Input: dimensioned drawing with shaded views. Units: mm. Origin: part minimum x, y, z. Coordinates: 2 decimals unless noted, no trailing zeros. Loops run counter-clockwise (first coordinate to the right, second up) from the corner with the lowest first, then second, coordinate; pieces in that order, holes last. Notation, with made-up numbers: (61, -32.5) - (93, -32.5) arc R22 cw to (93, -10.5) - close; hole circle Ø11 at (-1.75, 70). An arc over 180 degrees is marked (long way). Use one line per item in the form item = value. Start each with the question number.
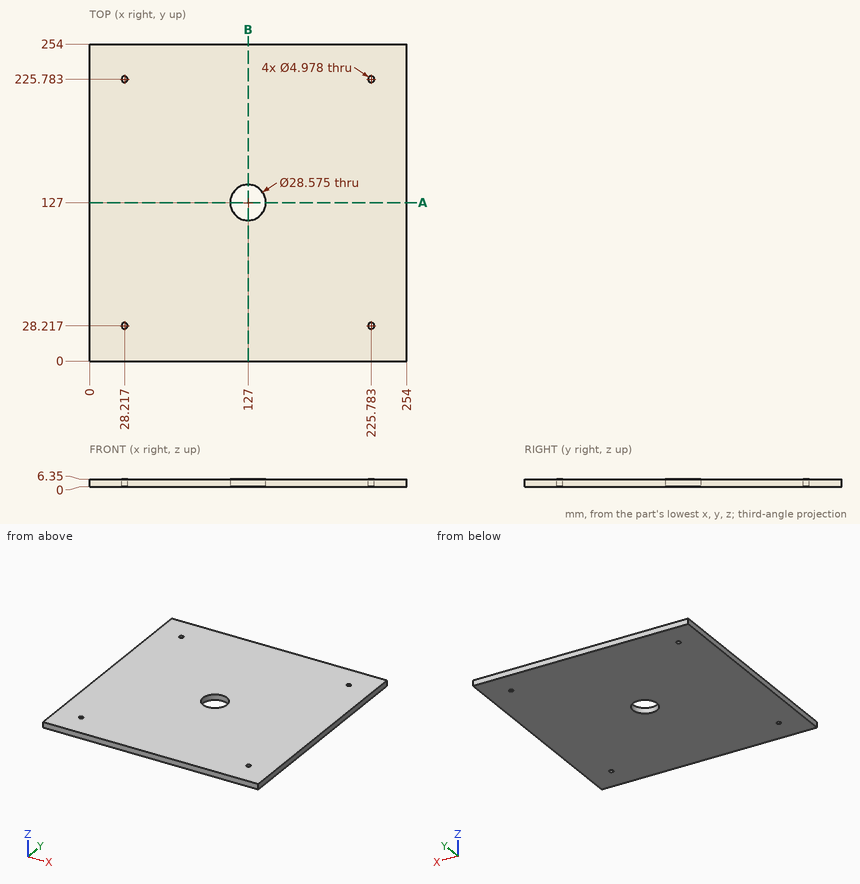
(1) Contact query for a flat-ended pin moving along its axis: pin 1 (3 mm diameter, centred on x = 28.22, y = 28.22, fed in from +Z). Output: stop coordinate, or through.
(2) Material intervals for line 1 (Y direction, x = 28, z = 5.25); line 2 (X direction, y = 138, z = 4) (1 decimal), sorted ascending.
(3) Cut plane A-A, the plane y = 127. Output: boundary loops of the cut face in (x, z), plus the area to 3 significant figures.
Recorded:
q1.pin_1 = through
q2.line_1 = 0 to 25.74, 30.7 to 223.3, 228.26 to 254
q2.line_2 = 0 to 117.9, 136.1 to 254
q3.outline = (0, 0) - (112.71, 0) - (112.71, 6.35) - (0, 6.35) - close; (141.29, 0) - (254, 0) - (254, 6.35) - (141.29, 6.35) - close
q3.area = 1,430 mm²
